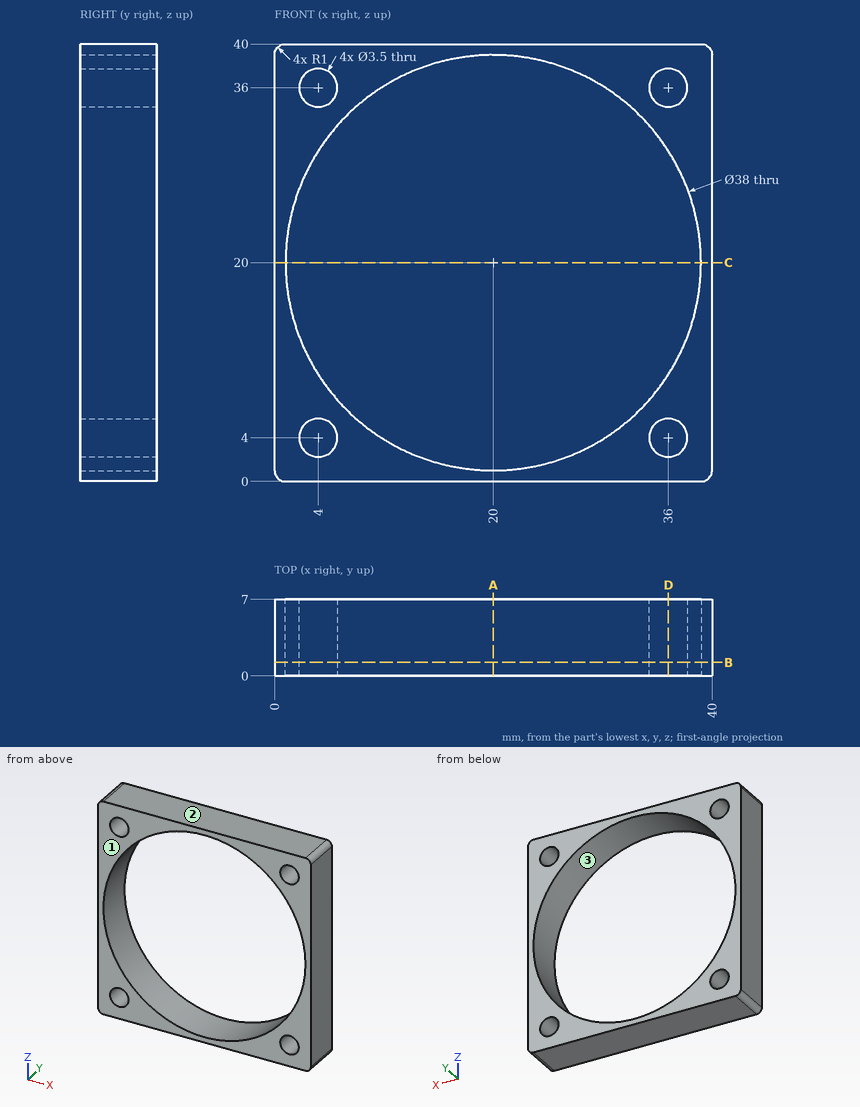
Could you check a few things on this drawing? It's one solid part, dimensions in mm from its lowest x, y, z. Coordinates: 2 decimals unless noted, no trailing zeros. Loops run counter-clockwise (first coordinate to the right, second up) from the corner with the lowest first, then second, coordinate; pieces in that order, holes last.
1. Imagine slicing it at C-C (z = 20). Please give me the cut outline in (x, y), and give its area (3 significant figures).
2. Imagine slicing it at A-A (x = 20). Please give me the cut outline in (y, z), and give its area (3 significant figures).
3. Imagine slicing it at D-D (x = 36). Please give me the cut outline in (y, z).
4. For P1, Ø10, axis at x = 18, z = 29.5, coming from the -Y side, with a flat end and sliding along its axis, tell me the tip position at first contact or that it passes through.
5. We'd pull the mould along Z, two halves only. Please class the marked faces 1, 2 and 3: released by +Z, released by -Z, zero draft, split by the parting line, or undercut.
6. Imagine slicing it at B-B (y = 1.25). Please give me the cut outline in (x, z), and give its area (3 significant figures).
7. I need wall thicknesses on L1, parallel to Z at x = 4, y = 5; L2, parallel to X at y = 2, z = 3.5; L3, parallel to Z at x = 19, y = 5.25. Which ranges of each line are inside material? Lowest first, please.
Computed values:
1. outline: (0, 0) - (1, 0) - (1, 7) - (0, 7) - close; (39, 0) - (40, 0) - (40, 7) - (39, 7) - close
1. area: 14.0 mm2
2. outline: (0, 0) - (7, 0) - (7, 1) - (0, 1) - close; (0, 39) - (7, 39) - (7, 40) - (0, 40) - close
2. area: 14.0 mm2
3. outline: (0, 0) - (7, 0) - (7, 2.25) - (0, 2.25) - close; (0, 5.75) - (7, 5.75) - (7, 9.75) - (0, 9.75) - close; (0, 30.25) - (7, 30.25) - (7, 34.25) - (0, 34.25) - close; (0, 37.75) - (7, 37.75) - (7, 40) - (0, 40) - close
4. P1: passes through
5. face 1: zero draft
5. face 2: released by +Z
5. face 3: undercut
6. outline: (0, 1) arc R1 ccw to (1, 0) - (39, 0) arc R1 ccw to (40, 1) - (40, 39) arc R1 ccw to (39, 40) - (1, 40) arc R1 ccw to (0, 39) - close; hole circle Ø38 at (20, 20); hole circle Ø3.5 at (4, 4); hole circle Ø3.5 at (4, 36); hole circle Ø3.5 at (36, 4); hole circle Ø3.5 at (36, 36)
6. area: 427 mm2
7. L1: z = 0 to 2.25, 5.75 to 9.75, 30.25 to 34.25, 37.75 to 40
7. L2: x = 0 to 2.32, 5.68 to 10.58, 29.42 to 34.32, 37.68 to 40
7. L3: z = 0 to 1.03, 38.97 to 40
